Part model, mm, in its own coordinate system. A direction names the side the tool comes from. Coordinates: 2 decimals unless noted, no trailing zeros. Order: outer loops, then holes, each group sorted by start corner. A loop starts at its lowest first (then second) coordinate and runs counter-clockwise, first axis right, second up.
1) Cut at C-C (z = 4). List the corners of the cut face in (x, y), and give its area (3 significant figures).
2) Mould opens along X. For faces 5 (the flat face through (12.23, 32.213, -3.594)), 6 (the flat face through (0, 242, 3)), 7 (the flat face through (17.74, 105.67, 4.93)) say: +X half, -X half, draft (parallel to the pull), parting line (faces both ways), or undercut.
3) Cut at D-D (y = 75.5). List the corners of the cut face in (x, z), and give its area (3 significant figures).
4) Cut at B-B (x = 13). List the corners of the cut face in (y, z), and give its area (3 significant figures).
5) Wall check: L1, parallel to Y at x = 9.5, z = -5.75; L2, parallel to Y at x = -15, z = -2; L3, parallel to Z at x = -29, y = 46. Give the ranges that are in metal, low to high.
6) Cut at A-A (y = 45). List the corners of the cut face in (x, z).
7) Pin check, flat tips, straight feed: pin 1 Ø6 at (x, z) = (28, -3.5) entering from +Y; pin 2 Ø8 at (x, z) = (8, 6) entering from +Y. Stop position of each tip, or through.
8) Tool access for faces 1 (the flat face through (-12.21, 222.28, 3.39)), 2 (the flat face through (-12.578, 32.213, -3.494)), 3 (the flat face through (-11.87, 222.28, -3.49)), 4 (the flat face through (12.21, 222.28, -3.39)): list every direction of +Z, -Z, +X, -X, +Y, -Y with a clear straight run to the whole face (end or side of a thin tool).
```python
from build123d import *

# Parameters (mm, degrees)
SWEEP_1_DEPTH            = 610
CUT_EXTRUDE_2_DEPTH      = 12
SKETCH_21_R              = 1.75
CUT_EXTRUDE_3_DEPTH      = 600
CUT_EXTRUDE_4_DEPTH      = 691.959477934
CUT_EXTRUDE_4_DEPTH_BACK = 691.959477934
SKETCH_26_OUTSIDE_W      = 208.38
SKETCH_26_OUTSIDE_H      = 816.38
SKETCH_26_OUTSIDE_W_2    = 70
SKETCH_26_OUTSIDE_H_2    = 230
CUT_EXTRUDE_5_DEPTH      = 41
SKETCH_28_OUTSIDE_W      = 120.25
SKETCH_28_OUTSIDE_H      = 70.25
CUT_EXTRUDE_7_DEPTH      = 40


# Read off the part's stored shape, not the designer's step: 扫描1
with BuildPart() as part:
    # 扫描1 outline → 扫描1 (new body)
    with BuildSketch(Plane(origin=(0, 0, 0), x_dir=(1, 0, 0), z_dir=(0, 1, 0))):
        Polygon((-35, 0), (35, 0), (0, 10), align=None)
    sweep_1 = extrude(amount=SWEEP_1_DEPTH)

    # 草图1 → 放样1 section 0
    with BuildSketch(Plane.XY, mode=Mode.PRIVATE) as loft_1_s0:
        with BuildLine():
            Line((-35, 610), (0, 690))
            Line((0, 690), (35, 610))
            Line((35, 610), (-35, 610))
        make_face()
    loft_1 = loft([Vertex(0, 610, -10), loft_1_s0.sketch])

    # 镜向1: 扫描1, 放样1 across plane
    add(sweep_1.mirror(Plane.XY))
    add(loft_1.mirror(Plane.XY))

    # 草图19 → 切除-拉伸2 (cut)
    with BuildSketch(Plane.XZ):
        Polygon((0, -10), (35, 0), (0, 10), (-35, 0), align=None)
    extrude(amount=-CUT_EXTRUDE_2_DEPTH, mode=Mode.SUBTRACT)

    # 草图21 → 切除-拉伸3 (cut)
    with BuildSketch(Plane.XZ.offset(-12)):
        with Locations(Location((0, 0, 0), (0, 0, 270))):
            Circle(SKETCH_21_R)
    extrude(amount=-CUT_EXTRUDE_3_DEPTH, mode=Mode.SUBTRACT)

    # 草图26 outside → 切除-拉伸4 (cut, two sides: drawn at the far end of the back side and taken through both)
    with BuildSketch(Plane.XY.offset(-CUT_EXTRUDE_4_DEPTH_BACK)):
        with Locations((0, 351)):
            Rectangle(SKETCH_26_OUTSIDE_W, SKETCH_26_OUTSIDE_H)
        with Locations((0, 127)):
            Rectangle(SKETCH_26_OUTSIDE_W_2, SKETCH_26_OUTSIDE_H_2, mode=Mode.SUBTRACT)
    extrude(amount=CUT_EXTRUDE_4_DEPTH + CUT_EXTRUDE_4_DEPTH_BACK, mode=Mode.SUBTRACT)

    # 草图27 → 切除-拉伸5 (cut)
    with BuildSketch(Plane.XZ.offset(-12)):
        Polygon((-24.807846155, 0), (0, -7.087956044), (24.807846155, 0), (0, 7.087956044), align=None)
    extrude(amount=-CUT_EXTRUDE_5_DEPTH, mode=Mode.SUBTRACT)

    # 草图28 outside → 切除-拉伸7 (cut)
    with BuildSketch(Plane(origin=(0, 242, 0), x_dir=(1, 0, 0), z_dir=(0, 1, 0))):
        Rectangle(SKETCH_28_OUTSIDE_W, SKETCH_28_OUTSIDE_H)
        Polygon((0, 6.879952905), (-24.079835166, 0), (0, -6.879952905), (24.079835166, 0), align=None, mode=Mode.SUBTRACT)
    extrude(amount=-CUT_EXTRUDE_7_DEPTH, mode=Mode.SUBTRACT)


solid = part.part
```
Geometry check:
1. outline: (-21, 12) - (-10.81, 12) - (-10.81, 53) - (10.81, 53) - (10.81, 12) - (21, 12) - (21, 202) - (10.08, 202) - (10.08, 242) - (-10.08, 242) - (-10.08, 202) - (-21, 202) - close
1. area: 7,900 mm2
2. face 5: undercut
2. face 6: draft
2. face 7: +X half
3. outline: (-35, 0) - (0, -10) - (35, 0) - (0, 10) - close; hole circle Ø3.5 at (0, 0)
3. area: 690 mm2
4. outline: (12, -6.29) - (202, -6.29) - (202, -3.17) - (242, -3.17) - (242, 3.17) - (202, 3.17) - (202, 6.29) - (12, 6.29) - (12, 3.37) - (53, 3.37) - (53, -3.37) - (12, -3.37) - close
4. area: 2,370 mm2
5. L1: y = 12 to 202
5. L2: y = 53 to 242
5. L3: z = -1.71 to 1.71
6. outline: (-35, 0) - (0, -10) - (35, 0) - (0, 10) - close; hole (-24.81, 0) - (0, -7.09) - (24.81, 0) - (0, 7.09) - close
7. pin 1: stops at y = 202
7. pin 2: stops at y = 242
8. face 1: +Z, -X, +Y
8. face 2: -Y
8. face 3: -Z, -X, +Y
8. face 4: -Z, +X, +Y
